```python
from build123d import *

# Parameters (mm, degrees)
BOSS_EXTRU_1_DEPTH      = 34
ENL_V_MAT_EXTRU_1_DEPTH = 32.5
ENL_V_MAT_EXTRU_2_REACH = 36
ESQUISSE3_R             = 2.75
BOSS_EXTRU_2_DEPTH      = 1
ESQUISSE5_R             = 3.4
ENL_V_MAT_EXTRU_3_DEPTH = 25
ESQUISSE6_R             = 3.5
ESQUISSE6_R_2           = 1.25
ESQUISSE6_R_3           = 2.1
BOSS_EXTRU_3_DEPTH      = 4.85
ENL_V_MAT_EXTRU_4_REACH = 101
ESQUISSE7_R             = 8


with BuildPart() as part:
    # Esquisse1 → Boss.-Extru.1 (new body)
    with BuildSketch(Plane(origin=(0, 0, 0), x_dir=(1, 0, 0), z_dir=(0, 1, 0))):
        with BuildLine():
            Line((-44.5, 34), (44.5, 34))
            ThreePointArc((44.5, 34), (48.035533906, 32.535533906), (49.5, 29))
            Line((49.5, 29), (49.5, -29))
            ThreePointArc((49.5, -29), (48.035533906, -32.535533906), (44.5, -34))
            Line((44.5, -34), (-44.5, -34))
            ThreePointArc((-44.5, -34), (-48.035533906, -32.535533906), (-49.5, -29))
            Line((-49.5, -29), (-49.5, 29))
            ThreePointArc((-49.5, 29), (-48.035533906, 32.535533906), (-44.5, 34))
        make_face()
    extrude(amount=BOSS_EXTRU_1_DEPTH)

    # Esquisse2 → Enlèv. mat.-Extru.1 (cut)
    with BuildSketch(Plane(origin=(0, 34, 0), x_dir=(1, 0, 0), z_dir=(0, 1, 0))):
        with BuildLine():
            Line((-36.5, 31), (36.5, 31))
            ThreePointArc((36.5, 31), (37.914213562, 30.414213562), (38.5, 29))
            ThreePointArc((38.5, 29), (40.257359313, 24.757359313), (44.5, 23))
            ThreePointArc((44.5, 23), (45.914213562, 22.414213562), (46.5, 21))
            Line((46.5, 21), (46.5, -21))
            ThreePointArc((46.5, -21), (45.914213562, -22.414213562), (44.5, -23))
            ThreePointArc((44.5, -23), (40.257359313, -24.757359313), (38.5, -29))
            ThreePointArc((38.5, -29), (37.914213562, -30.414213562), (36.5, -31))
            Line((36.5, -31), (-36.5, -31))
            ThreePointArc((-36.5, -31), (-37.914213562, -30.414213562), (-38.5, -29))
            ThreePointArc((-38.5, -29), (-40.257359313, -24.757359313), (-44.5, -23))
            ThreePointArc((-44.5, -23), (-45.914213562, -22.414213562), (-46.5, -21))
            Line((-46.5, -21), (-46.5, 21))
            ThreePointArc((-46.5, 21), (-45.914213562, 22.414213562), (-44.5, 23))
            ThreePointArc((-44.5, 23), (-40.257359313, 24.757359313), (-38.5, 29))
            ThreePointArc((-38.5, 29), (-37.914213562, 30.414213562), (-36.5, 31))
        make_face()
    extrude(amount=-ENL_V_MAT_EXTRU_1_DEPTH, mode=Mode.SUBTRACT)

    # Esquisse3 → Enlèv. mat.-Extru.2 (cut, up to next)
    with BuildSketch(Plane(origin=(0, 34, 0), x_dir=(1, 0, 0), z_dir=(0, 1, 0)), mode=Mode.PRIVATE) as enl_v_mat_extru_2_sk1:
        with Locations(Location((-44, 28, 0), (0, 0, 270))):  # turned: the seam where the file's is
            Circle(ESQUISSE3_R)
    enl_v_mat_extru_2_tool1 = extrude(enl_v_mat_extru_2_sk1.sketch, amount=-ENL_V_MAT_EXTRU_2_REACH, mode=Mode.PRIVATE) & part.part
    add(enl_v_mat_extru_2_tool1.solids().sort_by_distance((-44, 34, -28))[0], mode=Mode.SUBTRACT)
    # Esquisse3 → Enlèv. mat.-Extru.2 (cut, up to next)
    with BuildSketch(Plane(origin=(0, 34, 0), x_dir=(1, 0, 0), z_dir=(0, 1, 0)), mode=Mode.PRIVATE) as enl_v_mat_extru_2_sk2:
        with Locations(Location((-44, -28, 0), (0, 0, 270))):  # turned: the seam where the file's is
            Circle(ESQUISSE3_R)
    enl_v_mat_extru_2_tool2 = extrude(enl_v_mat_extru_2_sk2.sketch, amount=-ENL_V_MAT_EXTRU_2_REACH, mode=Mode.PRIVATE) & part.part
    add(enl_v_mat_extru_2_tool2.solids().sort_by_distance((-44, 34, 28))[0], mode=Mode.SUBTRACT)
    # Esquisse3 → Enlèv. mat.-Extru.2 (cut, up to next)
    with BuildSketch(Plane(origin=(0, 34, 0), x_dir=(1, 0, 0), z_dir=(0, 1, 0)), mode=Mode.PRIVATE) as enl_v_mat_extru_2_sk3:
        with Locations(Location((44, -28, 0), (0, 0, 270))):  # turned: the seam where the file's is
            Circle(ESQUISSE3_R)
    enl_v_mat_extru_2_tool3 = extrude(enl_v_mat_extru_2_sk3.sketch, amount=-ENL_V_MAT_EXTRU_2_REACH, mode=Mode.PRIVATE) & part.part
    add(enl_v_mat_extru_2_tool3.solids().sort_by_distance((44, 34, 28))[0], mode=Mode.SUBTRACT)
    # Esquisse3 → Enlèv. mat.-Extru.2 (cut, up to next)
    with BuildSketch(Plane(origin=(0, 34, 0), x_dir=(1, 0, 0), z_dir=(0, 1, 0)), mode=Mode.PRIVATE) as enl_v_mat_extru_2_sk4:
        with Locations(Location((44, 28, 0), (0, 0, 270))):  # turned: the seam where the file's is
            Circle(ESQUISSE3_R)
    enl_v_mat_extru_2_tool4 = extrude(enl_v_mat_extru_2_sk4.sketch, amount=-ENL_V_MAT_EXTRU_2_REACH, mode=Mode.PRIVATE) & part.part
    add(enl_v_mat_extru_2_tool4.solids().sort_by_distance((44, 34, -28))[0], mode=Mode.SUBTRACT)

    # Esquisse4 → Boss.-Extru.2 (add)
    with BuildSketch(Plane(origin=(0, 34, 0), x_dir=(1, 0, 0), z_dir=(0, 1, 0))):
        with BuildLine():
            Line((47.5, -21), (47.5, 21))
            ThreePointArc((47.5, 21), (46.621320344, 23.121320344), (44.5, 24))
            ThreePointArc((44.5, 24), (40.964466094, 25.464466094), (39.5, 29))
            ThreePointArc((39.5, 29), (38.621320344, 31.121320344), (36.5, 32))
            Line((36.5, 32), (-36.5, 32))
            ThreePointArc((-36.5, 32), (-38.621320344, 31.121320344), (-39.5, 29))
            ThreePointArc((-39.5, 29), (-40.964466094, 25.464466094), (-44.5, 24))
            ThreePointArc((-44.5, 24), (-46.621320344, 23.121320344), (-47.5, 21))
            Line((-47.5, 21), (-47.5, -21))
            ThreePointArc((-47.5, -21), (-46.621320344, -23.121320344), (-44.5, -24))
            ThreePointArc((-44.5, -24), (-40.964466094, -25.464466094), (-39.5, -29))
            ThreePointArc((-39.5, -29), (-38.621320344, -31.121320344), (-36.5, -32))
            Line((-36.5, -32), (36.5, -32))
            ThreePointArc((36.5, -32), (38.621320344, -31.121320344), (39.5, -29))
            ThreePointArc((39.5, -29), (40.964466094, -25.464466094), (44.5, -24))
            ThreePointArc((44.5, -24), (46.621320344, -23.121320344), (47.5, -21))
        make_face()
        with BuildLine():
            Line((46.5, -21), (46.5, 21))
            ThreePointArc((46.5, 21), (45.914213562, 22.414213562), (44.5, 23))
            ThreePointArc((44.5, 23), (40.257359313, 24.757359313), (38.5, 29))
            ThreePointArc((38.5, 29), (37.914213562, 30.414213562), (36.5, 31))
            Line((36.5, 31), (-36.5, 31))
            ThreePointArc((-36.5, 31), (-37.914213562, 30.414213562), (-38.5, 29))
            ThreePointArc((-38.5, 29), (-40.257359313, 24.757359313), (-44.5, 23))
            ThreePointArc((-44.5, 23), (-45.914213562, 22.414213562), (-46.5, 21))
            Line((-46.5, 21), (-46.5, -21))
            ThreePointArc((-46.5, -21), (-45.914213562, -22.414213562), (-44.5, -23))
            ThreePointArc((-44.5, -23), (-40.257359313, -24.757359313), (-38.5, -29))
            ThreePointArc((-38.5, -29), (-37.914213562, -30.414213562), (-36.5, -31))
            Line((-36.5, -31), (36.5, -31))
            ThreePointArc((36.5, -31), (37.914213562, -30.414213562), (38.5, -29))
            ThreePointArc((38.5, -29), (40.257359313, -24.757359313), (44.5, -23))
            ThreePointArc((44.5, -23), (45.914213562, -22.414213562), (46.5, -21))
        make_face(mode=Mode.SUBTRACT)
    extrude(amount=BOSS_EXTRU_2_DEPTH)

    # Esquisse5 → Enlèv. mat.-Extru.3 (cut)
    with BuildSketch(Plane.XZ):
        with Locations(Location((-44, 28, 0), (0, 0, 270))):  # turned: the seam where the file's is
            Circle(ESQUISSE5_R)
        with Locations(Location((44, 28, 0), (0, 0, 270))):  # turned: the seam where the file's is
            Circle(ESQUISSE5_R)
        with Locations(Location((44, -28, 0), (0, 0, 270))):  # turned: the seam where the file's is
            Circle(ESQUISSE5_R)
        with Locations(Location((-44, -28, 0), (0, 0, 270))):  # turned: the seam where the file's is
            Circle(ESQUISSE5_R)
    extrude(amount=-ENL_V_MAT_EXTRU_3_DEPTH, mode=Mode.SUBTRACT)

    # Esquisse6 → Boss.-Extru.3 (add)
    with BuildSketch(Plane(origin=(0, 1.5, 0), x_dir=(1, 0, 0), z_dir=(0, 1, 0))):
        with Locations(Location((-22.5, 23, 0), (0, 0, 270))):  # turned: the seam where the file's is
            Circle(ESQUISSE6_R)
        with Locations(Location((-22.5, 23, 0), (0, 0, 270))):  # turned: the seam where the file's is
            Circle(ESQUISSE6_R_2, mode=Mode.SUBTRACT)
        with Locations(Location((-40, 0, 0), (0, 0, 270))):  # turned: the seam where the file's is
            Circle(ESQUISSE6_R)
        with Locations(Location((-40, 0, 0), (0, 0, 270))):  # turned: the seam where the file's is
            Circle(ESQUISSE6_R_2, mode=Mode.SUBTRACT)
        with Locations(Location((-35, 20, 0), (0, 0, 270))):  # turned: the seam where the file's is
            Circle(ESQUISSE6_R_3)
        with Locations(Location((35, 20, 0), (0, 0, 90))):  # turned: the seam where the file's is
            Circle(ESQUISSE6_R_3)
        with Locations(Location((40, 0, 0), (0, 0, 90))):  # turned: the seam where the file's is
            Circle(ESQUISSE6_R)
        with Locations(Location((40, 0, 0), (0, 0, 90))):  # turned: the seam where the file's is
            Circle(ESQUISSE6_R_2, mode=Mode.SUBTRACT)
        with Locations(Location((22.5, 23, 0), (0, 0, 90))):  # turned: the seam where the file's is
            Circle(ESQUISSE6_R)
        with Locations(Location((22.5, 23, 0), (0, 0, 90))):  # turned: the seam where the file's is
            Circle(ESQUISSE6_R_2, mode=Mode.SUBTRACT)
        with Locations(Location((22.5, -23, 0), (0, 0, 270))):  # turned: the seam where the file's is
            Circle(ESQUISSE6_R)
        with Locations(Location((22.5, -23, 0), (0, 0, 270))):  # turned: the seam where the file's is
            Circle(ESQUISSE6_R_2, mode=Mode.SUBTRACT)
        with Locations(Location((35, -20, 0), (0, 0, 270))):  # turned: the seam where the file's is
            Circle(ESQUISSE6_R_3)
        with Locations(Location((-35, -20, 0), (0, 0, 90))):  # turned: the seam where the file's is
            Circle(ESQUISSE6_R_3)
        with Locations(Location((-22.5, -23, 0), (0, 0, 90))):  # turned: the seam where the file's is
            Circle(ESQUISSE6_R)
        with Locations(Location((-22.5, -23, 0), (0, 0, 90))):  # turned: the seam where the file's is
            Circle(ESQUISSE6_R_2, mode=Mode.SUBTRACT)
    extrude(amount=BOSS_EXTRU_3_DEPTH)

    # Esquisse7 → Enlèv. mat.-Extru.4 (cut, up to next)
    with BuildSketch(Plane(origin=(49.5, 0, 0), x_dir=(0, 0, -1), z_dir=(1, 0, 0)), mode=Mode.PRIVATE) as enl_v_mat_extru_4_sk1:
        with Locations((0, 22)):
            Circle(ESQUISSE7_R)
    enl_v_mat_extru_4_tool1 = extrude(enl_v_mat_extru_4_sk1.sketch, amount=-ENL_V_MAT_EXTRU_4_REACH, mode=Mode.PRIVATE) & part.part
    add(enl_v_mat_extru_4_tool1.solids().sort_by_distance((49.5, 22, 0))[0], mode=Mode.SUBTRACT)


solid = part.part
```
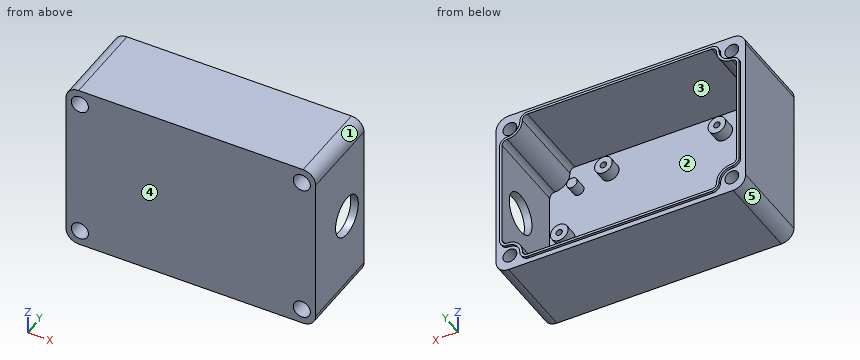
Verification items for the finished model (mm, model axes). Face numbers are marked on the shaded views. A direction names the side the tool comes from. Give positions to 0.01 mm unless a question says otherwise; leave off trailing zeros. Write each loop counter-clockwise with the first axis right and the second up, starting at its lowest first coordinate (ties: lowest second). Pieces come first, ordered by that corner, then holes. Notation, with made-up numbers: (0, 63.25) - (48, 63.25) arc R15 cw to (48, 74.25) - close; hole circle Ø1 at (89.25, -5). An arc over 180 degrees is marked (long way). Put each result on its own line as item: value.
Q1. Depth check by flat-ended pin: P1, Ø0.8, axis at x = 40.5, z = -0.5, coming from the +Y side; P2, Ø2, axis at y = 20, z = -6.5, coming from the +X side; P3, Ø4, axis at x = -22.5, z = 23, coming from the +Y side. Enter the tip coordinate at first touch or a pass-through.
Result:
P1: y = 1.5
P2: x = -46.5
P3: y = 6.35
Q2. Section check D-D on y = 22. Count the separate pieces of the cut face and the enclosed holes in it, and give its area (3 significant figures).
Result:
separate pieces: 1
enclosed holes: 4
area: 983 mm2
Q3. Scan lines: probe 1 along X at (y, z) = (5.1, 0); probe 2 along X at (y, z) = (4, -5); probe 3 along Z at (x, y) = (-24.5, 7). Record each from-to range of solid material in increasing order. Write a range as from..to.
Result:
probe 1: -49.5..-46.5, -43.5..-41.25, -38.75..-36.5, 36.5..38.75, 41.25..43.5, 46.5..49.5
probe 2: -49.5..-46.5, 46.5..49.5
probe 3: -34..-31, 31..34
Q4. Section check B-B on y = 32.5. Record the cut outline in (x, z), and give its area (3 significant figures).
Result:
outline: (-49.5, -29) arc R5 ccw to (-44.5, -34) - (44.5, -34) arc R5 ccw to (49.5, -29) - (49.5, 29) arc R5 ccw to (44.5, 34) - (-44.5, 34) arc R5 ccw to (-49.5, 29) - close; hole circle Ø5.5 at (-44, -28); hole circle Ø5.5 at (-44, 28); hole (-46.5, -21) arc R2 ccw to (-44.5, -23) arc R6 cw to (-38.5, -29) arc R2 ccw to (-36.5, -31) - (36.5, -31) arc R2 ccw to (38.5, -29) arc R6 cw to (44.5, -23) arc R2 ccw to (46.5, -21) - (46.5, 21) arc R2 ccw to (44.5, 23) arc R6 cw to (38.5, 29) arc R2 ccw to (36.5, 31) - (-36.5, 31) arc R2 ccw to (-38.5, 29) arc R6 cw to (-44.5, 23) arc R2 ccw to (-46.5, 21) - close; hole circle Ø5.5 at (44, -28); hole circle Ø5.5 at (44, 28)
area: 1,080 mm2
Q5. Set-up check for the marked faces 1 and 2: record each of +Z, -Z, +X, -X, +Y, -Y from which the full face is reachable in a straight line by a thin tool's end or side.
Result:
face 1: +Z, +X, +Y, -Y
face 2: +Y
Q6. Section check C-C on x = 35. Record the cut outline in (y, z), and give its area (3 significant figures).
Result:
outline: (0, -34) - (34, -34) - (34, -32) - (35, -32) - (35, -31) - (1.5, -31) - (1.5, -22.1) - (6.35, -22.1) - (6.35, -17.9) - (1.5, -17.9) - (1.5, 17.9) - (6.35, 17.9) - (6.35, 22.1) - (1.5, 22.1) - (1.5, 31) - (35, 31) - (35, 32) - (34, 32) - (34, 34) - (0, 34) - close
area: 340 mm2
Q7. Mould release check, pull along X, two halves, no side actions. Record for the marked faces 3, 4 and 5: released by +X, released by -X, zero draft, split by the parting line, or undercut.
Result:
face 3: undercut
face 4: zero draft
face 5: released by -X
